Autodesk Inventor part; units mm, degrees
ref_plane "part2a_XY" through (0, 0, 0) normal (0, 0, 1) x (1, 0, 0)
ref_plane "part2a_YZ" through (0, 0, 0) normal (1, 0, 0) x (0, 1, 0)
ref_plane "part2a_ZX" through (0, 0, 0) normal (0, 1, 0) x (0, 0, 1)
sketch "Sketch_1" plane through (0, 0, 0) normal (0, 0, 1) x (1, 0, 0)
  arc A0 (-13.4651, -6.61) -> (-6.61, -13.4651) centre (0, 0) ccw
  arc A1 (-6.61, -13.4651) -> (-1.6525, -7.3157) centre (-17.0197, 0) ccw
  arc A2 (-1.6525, -7.3157) -> (1.6525, -7.3157) centre (0, 0) ccw
  arc A3 (1.6525, -7.3157) -> (6.61, -13.4651) centre (17.0197, 0) ccw
  arc A4 (6.61, -13.4651) -> (13.4651, -6.61) centre (0, 0) ccw
  arc A5 (13.4651, -6.61) -> (7.3157, -1.6525) centre (0, -17.0197) ccw
  arc A6 (7.3157, -1.6525) -> (7.3157, 1.6525) centre (0, 0) ccw
  arc A7 (7.3157, 1.6525) -> (13.4651, 6.61) centre (0, 17.0197) ccw
  arc A8 (13.4651, 6.61) -> (6.61, 13.4651) centre (0, 0) ccw
  arc A9 (6.61, 13.4651) -> (1.6525, 7.3157) centre (17.0197, 0) ccw
  arc A10 (1.6525, 7.3157) -> (-1.6525, 7.3157) centre (0, 0) ccw
  arc A11 (-1.6525, 7.3157) -> (-6.61, 13.4651) centre (-17.0197, 0) ccw
  arc A12 (-6.61, 13.4651) -> (-13.4651, 6.61) centre (0, 0) ccw
  arc A13 (-13.4651, 6.61) -> (-7.3157, 1.6525) centre (0, 17.0197) ccw
  arc A14 (-7.3157, 1.6525) -> (-7.3157, -1.6525) centre (0, 0) ccw
  arc A15 (-7.3157, -1.6525) -> (-13.4651, -6.61) centre (0, -17.0197) ccw
extrude "Extrusion1" add sketch "Sketch_1" along normal blind 10
ref_plane "part2a_XY" through (0, 0, 0) normal (0, 0, 1) x (1, 0, 0)
ref_plane "part2a_YZ" through (0, 0, 0) normal (1, 0, 0) x (0, 1, 0)
ref_plane "part2a_ZX" through (0, 0, 0) normal (0, 1, 0) x (0, 0, 1)
properties part number "MJT-30-BL Sleeve"
Read the model definition and answer for the solid it produces. Units are mm, in the model's axes. A direction names the side the tool comes from. Coordinates: 2 decimals unless noted, no trailing zeros. Order: outer loops, then holes, each group sorted by start corner. A loop starts at its lowest first (then second) coordinate and runs counter-clockwise, first axis right, second up. Notation, with made-up numbers: (10.25, 50.5) - (25.25, 50.5) arc R12 cw to (25.25, 69.5) - close; hole circle Ø9 at (21, 47). An arc over 180 degrees is marked (long way). Answer as a JSON object with one key per item and string values. Group by question number.
Item 1: Consider probe 1 along Y at (x, z) = (9, 5.25); probe 2 along X at (y, z) = (11.75, 3.5); probe 3 along Y at (x, z) = (-10, 6.25). Determine where each line is inside the solid, lowest interval first. Write a range as from..to.
Item 2: Flat-ended cylindrical pins translate along their axes: P1, Ø4, axis at y = 2.5, z = 4.5, coming from the +X side; P2, Ø4, axis at x = -1.5, z = 8, coming from the -Y side; P3, Ø1, axis at x = 5.5, z = 6, coming from the +Y side. Find the tip coordinate at first contact, or state that the pin passes through.
Item 3: Section A-A (y = 9.5) is taken. Give the vertices of the cut face in (x, z).
Item 4: Section D-D (y = -4.75) is taken. Give the vertices of the cut face in (x, z), plus the area to 3 significant figures.
Item 5: Section C-C (x = 8) is taken. Give the vertices of the cut face in (y, z).
Item 6: The mould has two halves that part along Y. Classify faces 4 (the face through (10.725, 3.805, 4.93)), 5 (the face through (0, -7.5, 4.9)), 6 (the face through (0, 0, 0)): +Y half, -Y half, draft (parallel to the pull), parting line (faces both ways), or undercut.
Item 7: A tool of negligible diameter and unlimited length cuts with its end or side. For faces 1 (the face through (10.638, -3.735, 4.93)), 2 (the face through (-10.725, -3.805, 4.93)), 3 (the face through (-3.805, 10.725, 4.93)), from which of +Z, -Z, +X, -X, +Y, -Y can it reach the whole face along a straight path? Write none if from no direction.
Item 8: Section B-B (z = 7) is taken. Give the vertices of the cut face in (x, y).
Results are:
{
 "1": {"probe 1": "y = -12..-2.57, 2.57..12", "probe 2": "x = -9.32..-4.71, 4.71..9.32", "probe 3": "y = -11.18..-3.25, 3.25..11.18"},
 "2": {"P1": "stops at x = 11.53", "P2": "stops at y = -10.34", "P3": "stops at y = 12.97"},
 "3": {"outline": "(-11.61, 0) - (-2.9, 0) - (-2.9, 10) - (-11.61, 10) - close; (2.9, 0) - (11.61, 0) - (11.61, 10) - (2.9, 10) - close"},
 "4": {"outline": "(-11.8, 0) - (11.8, 0) - (11.8, 10) - (-11.8, 10) - close", "area": "236 mm^2"},
 "5": {"outline": "(-12.69, 0) - (-2, 0) - (-2, 10) - (-12.69, 10) - close; (2, 0) - (12.69, 0) - (12.69, 10) - (2, 10) - close"},
 "6": {"face 4": "undercut", "face 5": "-Y half", "face 6": "draft"},
 "7": {"face 1": "+Z, -Z, +X", "face 2": "+Z, -Z, -X", "face 3": "+Z, -Z, +Y"},
 "8": {"outline": "(-13.47, -6.61) arc R15 ccw to (-6.61, -13.47) arc R17.02 ccw to (-1.65, -7.32) arc R7.5 ccw to (1.65, -7.32) arc R17.02 ccw to (6.61, -13.47) arc R15 ccw to (13.47, -6.61) arc R17.02 ccw to (7.32, -1.65) arc R7.5 ccw to (7.32, 1.65) arc R17.02 ccw to (13.47, 6.61) arc R15 ccw to (6.61, 13.47) arc R17.02 ccw to (1.65, 7.32) arc R7.5 ccw to (-1.65, 7.32) arc R17.02 ccw to (-6.61, 13.47) arc R15 ccw to (-13.47, 6.61) arc R17.02 ccw to (-7.32, 1.65) arc R7.5 ccw to (-7.32, -1.65) arc R17.02 ccw to start"}
}
